```python
from build123d import *

# Parameters (mm, degrees)
SKETCH1_R           = 30
BOSS_EXTRUDE1_DEPTH = 25


with BuildPart() as part:
    # Sketch1 → Boss-Extrude1 (new body)
    with BuildSketch(Plane(origin=(0, 0, 0), x_dir=(1, 0, 0), z_dir=(0, 1, 0))):
        with BuildLine():
            Line((-108, 107), (-63.2, 107))
            ThreePointArc((-63.2, 107), (-31.521616203, 93.878383797), (-18.4, 62.2))
            Line((-18.4, 62.2), (-18.4, 53))
            ThreePointArc((-18.4, 53), (-14.885281374, 44.514718626), (-6.4, 41))
            Line((-6.4, 41), (0, 41))
            Line((0, 41), (6.4, 41))
            ThreePointArc((6.4, 41), (14.885281374, 44.514718626), (18.4, 53))
            Line((18.4, 53), (18.4, 62.2))
            ThreePointArc((18.4, 62.2), (31.521616203, 93.878383797), (63.2, 107))
            Line((63.2, 107), (108, 107))
            Line((108, 107), (108, 62.2))
            ThreePointArc((108, 62.2), (98.171988791, 34.2), (73, 18.485014011))
            Line((73, 18.485014011), (73, -18.485014011))
            ThreePointArc((73, -18.485014011), (98.171988791, -34.2), (108, -62.2))
            Line((108, -62.2), (108, -107))
            Line((108, -107), (63.2, -107))
            ThreePointArc((63.2, -107), (31.521616203, -93.878383797), (18.4, -62.2))
            Line((18.4, -62.2), (18.4, -53))
            ThreePointArc((18.4, -53), (14.885281374, -44.514718626), (6.4, -41))
            Line((6.4, -41), (0, -41))
            Line((0, -41), (-6.4, -41))
            ThreePointArc((-6.4, -41), (-14.885281374, -44.514718626), (-18.4, -53))
            Line((-18.4, -53), (-18.4, -62.2))
            ThreePointArc((-18.4, -62.2), (-31.521616203, -93.878383797), (-63.2, -107))
            Line((-63.2, -107), (-108, -107))
            Line((-108, -107), (-108, -62.2))
            ThreePointArc((-108, -62.2), (-98.171988791, -34.2), (-73, -18.485014011))
            Line((-73, -18.485014011), (-73, 18.485014011))
            ThreePointArc((-73, 18.485014011), (-98.171988791, 34.2), (-108, 62.2))
            Line((-108, 62.2), (-108, 107))
        make_face()
        with Locations(Location((0, 0, 0), (0, 0, 270))):
            Circle(SKETCH1_R, mode=Mode.SUBTRACT)
        with BuildLine():
            Line((-63.2, 94.7), (-95.7, 94.7))
            Line((-95.7, 94.7), (-95.7, 62.2))
            ThreePointArc((-95.7, 62.2), (-40.219029611, 39.219029611), (-63.2, 94.7))
        make_face(mode=Mode.SUBTRACT)
        with BuildLine():
            Line((-63.2, -94.7), (-95.7, -94.7))
            Line((-95.7, -94.7), (-95.7, -62.2))
            ThreePointArc((-95.7, -62.2), (-40.219029611, -39.219029611), (-63.2, -94.7))
        make_face(mode=Mode.SUBTRACT)
        with BuildLine():
            Line((63.2, -94.7), (95.7, -94.7))
            Line((95.7, -94.7), (95.7, -62.2))
            ThreePointArc((95.7, -62.2), (40.219029611, -39.219029611), (63.2, -94.7))
        make_face(mode=Mode.SUBTRACT)
        with BuildLine():
            Line((63.2, 94.7), (95.7, 94.7))
            Line((95.7, 94.7), (95.7, 62.2))
            ThreePointArc((95.7, 62.2), (40.219029611, 39.219029611), (63.2, 94.7))
        make_face(mode=Mode.SUBTRACT)
    extrude(amount=BOSS_EXTRUDE1_DEPTH)


solid = part.part
```
Can you work these out from the model? Positions are in its coordinate system, mm. A direction names the side the tool comes from. Give positions to 0.01 mm unless a question says otherwise; leave off trailing zeros. Write each loop counter-clockwise with the first axis right and the second up, starting at its lowest first coordinate (ties: lowest second). Pieces come first, ordered by that corner, then holes. Notation, with made-up numbers: (-5, -32) -> (16, -32) arc R16 ccw to (16, -6) -> close; hole circle Ø11 at (69, 82.25). An arc over 180 degrees is marked (long way). One line per item, written item: value.
Q1. We'd pull the mould along X, two halves only. Please class faces 4 (the face through (-31.872, 12.325, -94.225)), 5 (the face through (-97.906, 12.325, -33.871)), 6 (the face through (97.906, 12.325, 33.871)): +X half, -X half, draft (parallel to the pull), parting line (faces both ways), or undercut.
Results found:
face 4: undercut
face 5: -X half
face 6: +X half
Q2. Imagine slicing it at A-A on z = 0. Please give me the cut outline in (x, y).
Results found:
outline: (-73, 0) -> (-30, 0) -> (-30, 25) -> (-73, 25) -> close; (30, 0) -> (73, 0) -> (73, 25) -> (30, 25) -> close
Q3. Imagine slicing it at D-D on y = 8.5. Give the number of separate pieces and of enclosed holes in the cut face, and give its area (3 significant figures).
Results found:
separate pieces: 1
enclosed holes: 5
area: 18,600 mm^2
Q4. Which directions (+Z, -Z, +X, -X, +Y, -Y) give clear straight access to the entire face, cutting with the end or side of a thin tool? Please do faces 1 (the face through (-14.79, 12.32, 44.42)), 2 (the face through (18.4, 12, -58)), 3 (the face through (79, 12, -94.7)).
Results found:
face 1: +Z, +Y, -Y
face 2: -Z, +Y, -Y
face 3: +Y, -Y
Q5. For P1, Ø10, axis at x = -2.5, y = 8.5, coming from the +Z side; P2, Ø1, axis at x = -35, y = 3, coming from the -Z side; P3, Ø4.5, axis at y = 18.5, z = 57, coming from the -X side, each with a flat end and sliding along its axis, tell me the tip position at first contact or that it passes through.
Results found:
P1: stops at z = 41.05
P2: stops at z = -97.41
P3: stops at x = -107.9
Q6. Imagine slicing it at C-C on x = 36. Please give me the cut outline in (y, z), and give its area (3 significant figures).
Results found:
outline: (0, -97.8) -> (25, -97.8) -> (25, -79.99) -> (0, -79.99) -> close; (0, -44.41) -> (25, -44.41) -> (25, 44.41) -> (0, 44.41) -> close; (0, 79.99) -> (25, 79.99) -> (25, 97.8) -> (0, 97.8) -> close
area: 3,110 mm^2
Q7. Please list where these lines run through material, in increasing order: line 1 (X direction, y = 11.25, z = 62.2); line 2 (Z direction, x = 63.2, y = 19); line 3 (Z direction, x = 51, y = 19). Write a range as [from, to].
Results found:
line 1: x = [-108, -95.7], [-30.7, -18.4], [18.4, 30.7], [95.7, 108]
line 2: z = [-107, -94.7], [-29.7, 29.7], [94.7, 107]
line 3: z = [-105.31, -92.32], [-32.08, 32.08], [92.32, 105.31]
Q8. Imagine slicing it at B-B on x = 0. Please give me the cut outline in (y, z).
Results found:
outline: (0, -41) -> (25, -41) -> (25, -30) -> (0, -30) -> close; (0, 30) -> (25, 30) -> (25, 41) -> (0, 41) -> close
